Here's how the part is built. I have some questions about the finished solid (model axes, mm). Give positions to 0.01 mm unless a question says otherwise; leave off trailing zeros. Write each loop counter-clockwise with the first axis right and the second up, starting at its lowest first coordinate (ties: lowest second). Pieces come first, ordered by that corner, then holes. Notation, with made-up numbers: (49.25, 71) -> (72.25, 71) arc R4 ccw to (72.25, 78) -> close; hole circle Ø1 at (-22.75, 33.25). An arc over 180 degrees is marked (long way). Use one line per item in the form item = value.
```python
from build123d import *

# Parameters (mm, degrees)
F0_W      = 609.6
F0_H      = 609.6
F1_DEPTH  = 12.7
F2_R      = 12.065
F3_DEPTH  = 50.8
F7_DEPTH  = 266.7
F8_DEPTH  = 254
F9_DEPTH  = 165.1
F10_DEPTH = 152.4


with BuildPart() as f1:
    # F0 (on Top) → F1 (new body)
    with BuildSketch(Plane.XY):
        with Locations((304.8, 304.8)):
            Rectangle(F0_W, F0_H)
    extrude(amount=F1_DEPTH)

    # F2 (on face) → F3 (join)
    with BuildSketch(Plane(origin=(0, 0, 0), x_dir=(1, 0, 0), z_dir=(0, 0, -1))):
        with Locations((304.8, -304.8)):
            Circle(F2_R)
    extrude(amount=F3_DEPTH)

    # F6 (on offset) → F7 (join, symmetric)
    with BuildSketch(Plane.XZ.offset(-304.8)):
        with BuildLine():
            ThreePointArc((127.591476, 222.802752), (213.718068, 133.783712), (239.812403, 12.7))
            Line((239.812403, 12.7), (284.343503, 12.7))
            ThreePointArc((284.343503, 12.7), (252.229854, 156.01992), (149.816476, 261.297581))
            ThreePointArc((149.816476, 261.297581), (119.456561, 253.162667), (127.591476, 222.802752))
        make_face()
        with BuildLine():
            ThreePointArc((265.703976, 27.578975), (262.528976, 24.403975), (259.353976, 27.578975))
            ThreePointArc((259.353976, 27.578975), (226.600536, 149.816475), (137.116476, 239.300536))
            ThreePointArc((137.116476, 239.300536), (135.954345, 243.637667), (140.291476, 244.799797))
            ThreePointArc((140.291476, 244.799797), (232.099797, 152.991475), (265.703976, 27.578975))
        make_face(mode=Mode.SUBTRACT)
    extrude(amount=F7_DEPTH, both=True)

    # F6 (on offset) → F8 (cut, symmetric)
    with BuildSketch(Plane.XZ.offset(-304.8)):
        with BuildLine():
            ThreePointArc((127.591476, 222.802752), (213.718068, 133.783712), (239.812403, 12.7))
            Line((239.812403, 12.7), (284.343503, 12.7))
            ThreePointArc((284.343503, 12.7), (252.229854, 156.01992), (149.816476, 261.297581))
            ThreePointArc((149.816476, 261.297581), (119.456561, 253.162667), (127.591476, 222.802752))
        make_face()
        with BuildLine():
            ThreePointArc((265.703976, 27.578975), (262.528976, 24.403975), (259.353976, 27.578975))
            ThreePointArc((259.353976, 27.578975), (226.600536, 149.816475), (137.116476, 239.300536))
            ThreePointArc((137.116476, 239.300536), (135.954345, 243.637667), (140.291476, 244.799797))
            ThreePointArc((140.291476, 244.799797), (232.099797, 152.991475), (265.703976, 27.578975))
        make_face(mode=Mode.SUBTRACT)
    extrude(amount=F8_DEPTH, both=True, mode=Mode.SUBTRACT)

    # F5 (on offset) → F9 (join, symmetric)
    with BuildSketch(Plane.XZ.offset(-304.8)):
        with BuildLine():
            Line((0, 46.355), (0, 12.7))
            Line((0, 12.7), (23.1775, 12.7))
            ThreePointArc((23.1775, 12.7), (6.35, 29.5275), (23.1775, 46.355))
            Line((23.1775, 46.355), (0, 46.355))
        make_face()
    extrude(amount=F9_DEPTH, both=True)

    # F5 (on offset) → F10 (cut, symmetric)
    with BuildSketch(Plane.XZ.offset(-304.8)):
        with BuildLine():
            Line((0, 46.355), (0, 12.7))
            Line((0, 12.7), (23.1775, 12.7))
            ThreePointArc((23.1775, 12.7), (6.35, 29.5275), (23.1775, 46.355))
            Line((23.1775, 46.355), (0, 46.355))
        make_face()
    extrude(amount=F10_DEPTH, both=True, mode=Mode.SUBTRACT)


solid = f1.part
```
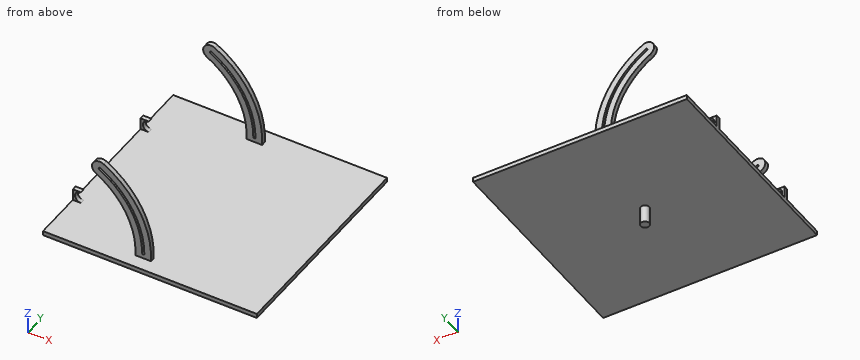
Q1. I want a section at C-C, the plane x = 203.5. Write out the boundary of the cut face in (y, z).
Result set:
outline = (0, 0) -> (609.6, 0) -> (609.6, 12.7) -> (0, 12.7) -> close; (38.1, 151.02) -> (50.8, 151.02) -> (50.8, 183.11) -> (38.1, 183.11) -> close; (38.1, 192.91) -> (50.8, 192.91) -> (50.8, 220.59) -> (38.1, 220.59) -> close; (558.8, 151.02) -> (571.5, 151.02) -> (571.5, 183.11) -> (558.8, 183.11) -> close; (558.8, 192.91) -> (571.5, 192.91) -> (571.5, 220.59) -> (558.8, 220.59) -> close
Q2. Will these pins go through, and if not, where does the flat tip stop? pin 1 Ø12 at (x, y) = (63, 393.5) entering from -Z; pin 2 Ø18.5 at (x, z) = (8.5, 23.5) entering from +Y; pin 3 Ø1.5 at (x, y) = (247.5, 245) entering from +Z.
Result set:
pin_1 = 0
pin_2 = 469.9
pin_3 = 12.7
Q3. If I drill on line 1 along Y through (x, z) = (183, 202.5); line 2 along Z through (x, y) = (306, 551), over which ranges is the centre line in solid material (lowest first)? Write a range as from..to.
Result set:
line_1 = 38.1..50.8, 558.8..571.5
line_2 = 0..12.7
Q4. I want a section at B-B, the plane y = 304.8. Write out the boundary of the cut face in (x, z) (3 decimals), and give its area (3 significant figures).
Result set:
outline = (0, 0) -> (292.735, 0) -> (292.735, -50.8) -> (316.865, -50.8) -> (316.865, 0) -> (609.6, 0) -> (609.6, 12.7) -> (0, 12.7) -> close
area = 8,970 mm2
Q5. I want a section at A-A, the plane z = 175. Write out the boundary of the cut face in (x, y).
Result set:
outline = (185.42, 38.1) -> (209.9, 38.1) -> (209.9, 50.8) -> (185.42, 50.8) -> close; (185.42, 558.8) -> (209.9, 558.8) -> (209.9, 571.5) -> (185.42, 571.5) -> close; (217.81, 38.1) -> (240.93, 38.1) -> (240.93, 50.8) -> (217.81, 50.8) -> close; (217.81, 558.8) -> (240.93, 558.8) -> (240.93, 571.5) -> (217.81, 571.5) -> close
